The listing builds one solid part. Answer for the finished solid, in the listing's coordinates (mm). A direction names the side the tool comes from. Give positions to 0.01 mm unless a question says otherwise; leave off trailing zeros. Write each loop counter-clockwise with the first axis right and the second up, starting at its lowest first coordinate (ties: lowest second). Pieces come first, ordered by that corner, then holes. Notation, with made-up numbers: (63, 58.25) - (75, 58.25) arc R23 ccw to (75, 68.25) - close; hole circle Ø10 at (-2, 14.25). An arc over 180 degrees is marked (long way). Answer as CSV lines item,"result". Start each with the question number.
(1) For faces 4 (the face through (-156.25, 7, 0)), 5 (the face through (2, -8, 0)), 6 (the face through (93.748, 12.972, -0.11)), determine the directions among +Z, -Z, +X, -X, +Y, -Y from which every point of the face is accessible in a straight line to the end or side of a thin tool.
(2) Each of these flat-tipped pins is pushed along its axis until it touches: pin 1 Ø1.5 at (x, z) = (41.5, 6) entering from +Y; pin 2 Ø1.5 at (x, y) = (45.5, -6.5) entering from -Z. Where does it stop, or does it pass through?
(3) Find section B-B (x = 1). State how many separate pieces and enclosed holes the cut face has, then the cut area to 3 significant figures.
(4) For a pull along Z with two mould halves and no side action, classify faces 1 (the face through (2, 12, -15)), 2 (the face through (103.865, 6.986, -0.751)), 3 (the face through (156.25, 7, 0)) as pulls with the +Z half, pulls with the -Z half, needs draft (parallel to the pull), parting line crosses it, or undercut.
(5) Straight lines are drawn through the part: probe 1 along Y at (x, z) = (-126, -7.5); probe 2 along Z at (x, y) = (106.25, 13.85); probe 3 along Y at (x, z) = (-121, -13). For each, find the intervals that lie inside material, in ascending order.
(6) Find section A-A (y = 1). Write down the section's boundary in (x, z).
from build123d import *

# Parameters (mm, degrees)
SKETCH_1_W             = 23.5
SKETCH_1_H             = 12
EXTRUDE_1_DEPTH        = 156.25
HOLE_WIZARD_M6_1_D     = 5
HOLE_WIZARD_M6_1_DEPTH = 19
HOLE_WIZARD_M6_1_TIP   = 1.502151548


with BuildPart() as part:
    # 草图1 → 凸台-拉伸1 (new, symmetric)
    with BuildSketch(Plane(origin=(0, 0, 0), x_dir=(0, 0, -1), z_dir=(1, 0, 0))):
        Polygon((-15, 15), (-11.5, 15), (-11.5, 13.5), (-11, 13.5), (-11, 12), (-9.5, 12), (-9.5, 15), (-8, 15), (-8, 12.5), (-5, 12.5), (-5, 15), (5, 15), (5, 12.5), (8, 12.5), (8, 15), (9.5, 15), (9.5, 12), (11, 12), (11, 13.5), (11.5, 13.5), (11.5, 15), (15, 15), (15, 8), (12.5, 8), (12.5, 5), (15, 5), (15, -5), (12.5, -5), (12.5, -8), (15, -8), (15, -15), (11.5, -15), (11.5, -13.5), (11, -13.5), (11, -12), (9.5, -12), (9.5, -15), (8, -15), (8, -12.5), (5, -12.5), (5, -15), (-5, -15), (-5, -12.5), (-8, -12.5), (-8, -15), (-9.5, -15), (-9.5, -12), (-11, -12), (-11, -13.5), (-11.5, -13.5), (-11.5, -15), (-15, -15), align=None)
        with BuildLine():
            Line((12, -10.5), (12, -8.5))
            ThreePointArc((12, -8.5), (11.853553391, -8.146446609), (11.5, -8))
            Line((11.5, -8), (-11.5, -8))
            ThreePointArc((-11.5, -8), (-11.853553391, -8.146446609), (-12, -8.5))
            Line((-12, -8.5), (-12, -10.5))
            ThreePointArc((-12, -10.5), (-11.853553391, -10.853553391), (-11.5, -11))
            Line((-11.5, -11), (11.5, -11))
            ThreePointArc((11.5, -11), (11.853553391, -10.853553391), (12, -10.5))
        make_face(mode=Mode.SUBTRACT)
        with BuildLine():
            Line((-11.5, 11), (11.5, 11))
            ThreePointArc((11.5, 11), (11.853553391, 10.853553391), (12, 10.5))
            Line((12, 10.5), (12, 8.5))
            ThreePointArc((12, 8.5), (11.853553391, 8.146446609), (11.5, 8))
            Line((11.5, 8), (-11.5, 8))
            ThreePointArc((-11.5, 8), (-11.853553391, 8.146446609), (-12, 8.5))
            Line((-12, 8.5), (-12, 10.5))
            ThreePointArc((-12, 10.5), (-11.853553391, 10.853553391), (-11.5, 11))
        make_face(mode=Mode.SUBTRACT)
        Rectangle(SKETCH_1_W, SKETCH_1_H, mode=Mode.SUBTRACT)
    extrude(amount=EXTRUDE_1_DEPTH, both=True)

    # M6 螺纹孔1
    with Locations(Plane(origin=(0, 15, 0), x_dir=(1, 0, 0), z_dir=(0, 1, 0))):
        with Locations((106.25, 0), (91.25, 0), (-121.25, 0), (-136.25, 0)):
            Hole(HOLE_WIZARD_M6_1_D / 2, depth=HOLE_WIZARD_M6_1_DEPTH)
            with Locations((0, 0, -(HOLE_WIZARD_M6_1_DEPTH + HOLE_WIZARD_M6_1_TIP / 2))):  # 118° drill point
                Cone(0, HOLE_WIZARD_M6_1_D / 2, HOLE_WIZARD_M6_1_TIP, mode=Mode.SUBTRACT)


solid = part.part
Result set:
1,face 4,"+Z, -Z, -X, +Y, -Y"
1,face 5,"+X, -X"
1,face 6,"+Y"
2,pin 1,"y = 12.5"
2,pin 2,"z = -12.5"
3,separate pieces,"1"
3,enclosed holes,"3"
3,area,"408 mm^2"
4,face 1,"pulls with the -Z half"
4,face 2,"undercut"
4,face 3,"needs draft"
5,probe 1,"-12.5 to -11, -8 to -6, 6 to 8, 11 to 12.5"
5,probe 2,"-15 to -11.5, -9.5 to -8, -5 to -2.5, 2.5 to 5, 8 to 9.5, 11.5 to 15"
5,probe 3,"-15 to -8, -5 to 5, 8 to 15"
6,outline,"(-156.25, -15) - (156.25, -15) - (156.25, -11.75) - (-156.25, -11.75) - close; (-156.25, 11.75) - (156.25, 11.75) - (156.25, 15) - (-156.25, 15) - close"
